Could you check a few things on this drawing? It's one solid part, dimensions in mm from its lowest x, y, z. A direction names the side the tool comes from. Give positions to 0.01 mm unless a question says otherwise; leave off trailing zeros. Order: outer loops, then holes, each group sorted by start corner. A loop starts at its lowest first (then second) coordinate and runs counter-clockwise, first axis right, second up. Notation, with made-up numbers: (82.25, -1.75) -> (141.25, -1.75) arc R35 ccw to (141.25, 32.25) -> close; hole circle Ø6 at (73, 75.25). An arc over 180 degrees is marked (long way). Answer as a JSON object with one key per item and string values.
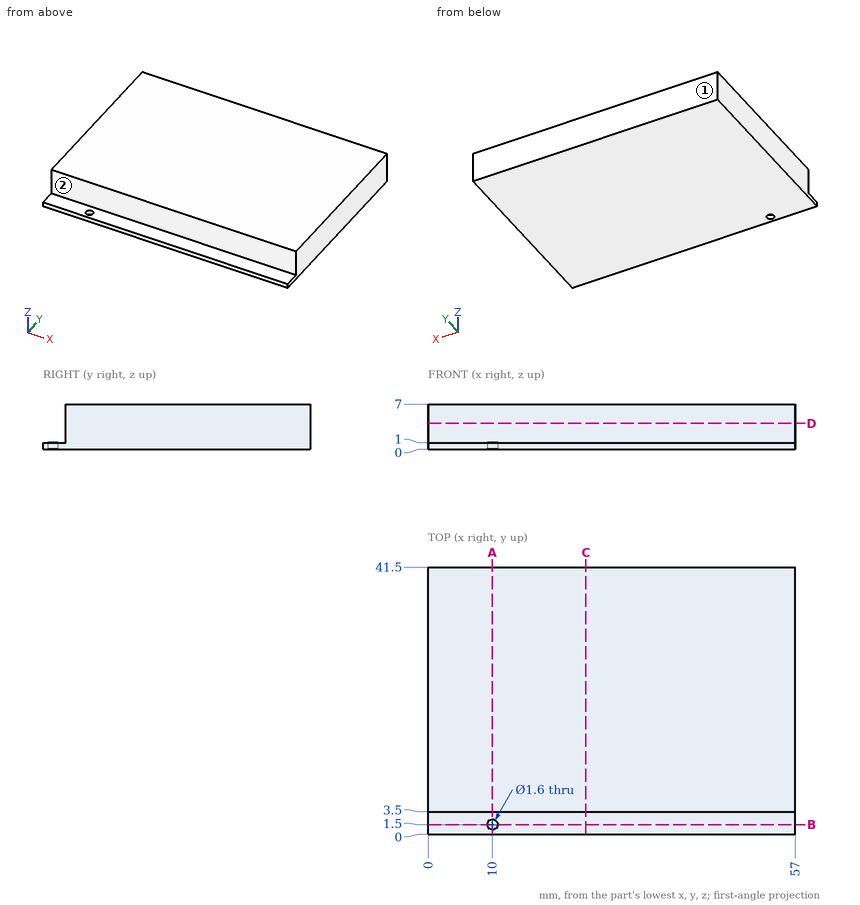
1. Please list where these lines run through material, in increasing order: L1, parallel to Y at x = 10, z = 0.3; L2, parallel to Y at x = 37, z = 2.5; L3, parallel to Z at x = 34.5, y = 2.
Worked answers:
{"L1": "0 to 0.7, 2.3 to 41.5", "L2": "3.5 to 41.5", "L3": "0 to 1"}
2. If we section it at B-B on y = 1.5: Please give me the cut outline in (x, z).
Worked answers:
{"outline": "(0, 0) -> (9.2, 0) -> (9.2, 1) -> (0, 1) -> close; (10.8, 0) -> (57, 0) -> (57, 1) -> (10.8, 1) -> close"}
3. Will these pins go through, and if not, where does the flat tip stop? pin 1 Ø2 at (x, y) = (10, 1.5) entering from +Z; pin 2 Ø4 at (x, z) = (14.5, 6) entering from -Y.
Worked answers:
{"pin 1": "z = 1", "pin 2": "y = 3.5"}
4. For the marked faces 1 and 2, which set-ups out of +Z, -Z, +X, -X, +Y, -Y let a thin tool reach every point of the face, with its end or its side?
Worked answers:
{"face 1": "+Z, -Z, +X, -X, +Y", "face 2": "+Z, +X, -X, -Y"}
5. If we section it at D-D on z = 4: Please give me the cut outline in (x, y).
Worked answers:
{"outline": "(0, 3.5) -> (57, 3.5) -> (57, 41.5) -> (0, 41.5) -> close"}
6. If we section it at C-C on x = 24.5: Please give me the cut outline in (y, z).
Worked answers:
{"outline": "(0, 0) -> (41.5, 0) -> (41.5, 7) -> (3.5, 7) -> (3.5, 1) -> (0, 1) -> close"}
7. If we section it at A-A on x = 10: Please give me the cut outline in (y, z).
Worked answers:
{"outline": "(0, 0) -> (0.7, 0) -> (0.7, 1) -> (0, 1) -> close; (2.3, 0) -> (41.5, 0) -> (41.5, 7) -> (3.5, 7) -> (3.5, 1) -> (2.3, 1) -> close"}
